from build123d import *

# Parameters (mm, degrees)
CROQUIS1_R                   = 25
CROQUIS1_R_2                 = 15
SALIENTE_EXTRUIR1_DEPTH      = 75
SALIENTE_EXTRUIR3_REACH      = 184.916
SALIENTE_EXTRUIR3_END_RADIUS = 25
SALIENTE_EXTRUIR3_START      = 100
CROQUIS2_R                   = 25
CROQUIS2_R_2                 = 15
CORTAR_EXTRUIR1_REACH        = 129.475
CROQUIS2_2_R                 = 15
SALIENTE_EXTRUIR4_REACH      = 164.475
SALIENTE_EXTRUIR4_END_RADIUS = 25
SALIENTE_EXTRUIR4_START      = 35
CROQUIS3_W                   = 35
CROQUIS3_H                   = 30
REDONDEO1_R                  = 15
CROQUIS4_R                   = 8
CORTAR_EXTRUIR2_DEPTH        = 151.7481344
SALIENTE_EXTRUIR5_START      = 55
SALIENTE_EXTRUIR5_DEPTH      = 10
SALIENTE_EXTRUIR6_START      = 22.912881
CROQUIS6_R                   = 10
CROQUIS6_R_2                 = 5
SALIENTE_EXTRUIR6_DEPTH      = 12.087119
CORTAR_EXTRUIR3_REACH        = 149.717
CROQUIS6_2_R                 = 5
REDONDEO1_OF_SIMETR_A1_R     = 15


with BuildPart() as part:
    # Croquis1 → Saliente-Extruir1 (new, symmetric)
    with BuildSketch(Plane.XY):
        Circle(CROQUIS1_R)
        Circle(CROQUIS1_R_2, mode=Mode.SUBTRACT)
    extrude(amount=SALIENTE_EXTRUIR1_DEPTH, both=True)

    # Saliente-Extruir3: up to this cylinder (the profile starts outside it)
    saliente_extruir3_end = Plane(origin=(0, 0, 24.292893), z_dir=(0, 0, -1)) * Cylinder(SALIENTE_EXTRUIR3_END_RADIUS, 420.832, mode=Mode.PRIVATE)
    # Croquis2 → Saliente-Extruir3 (add, up to the surface)
    with BuildSketch(Plane(origin=(0, 0, 0), x_dir=(0, 0, -1), z_dir=(1, 0, 0)).offset(SALIENTE_EXTRUIR3_START), mode=Mode.PRIVATE) as saliente_extruir3_sk1:
        Circle(CROQUIS2_R)
        Circle(CROQUIS2_R_2, mode=Mode.SUBTRACT)
    saliente_extruir3_tool1 = extrude(saliente_extruir3_sk1.sketch, amount=-SALIENTE_EXTRUIR3_REACH, mode=Mode.PRIVATE) - saliente_extruir3_end
    add(saliente_extruir3_tool1.solids().sort_by_distance((100, 0, 24.292893))[0])

    # Croquis2<2> → Cortar-Extruir1 (cut, up to next)
    with BuildSketch(Plane(origin=(0, 0, 0), x_dir=(0, 0, -1), z_dir=(1, 0, 0)), mode=Mode.PRIVATE) as cortar_extruir1_sk1:
        Circle(CROQUIS2_2_R)
    cortar_extruir1_tool1 = extrude(cortar_extruir1_sk1.sketch, amount=CORTAR_EXTRUIR1_REACH, mode=Mode.PRIVATE) & part.part
    add(cortar_extruir1_tool1.solids().sort_by_distance((0, 0, 0))[0], mode=Mode.SUBTRACT)

    # Saliente-Extruir4: up to this cylinder (the profile starts outside it)
    saliente_extruir4_end = Plane(origin=(82.5, 0, 0), z_dir=(1, 0, 0)) * Cylinder(SALIENTE_EXTRUIR4_END_RADIUS, 379.95, mode=Mode.PRIVATE)
    # Croquis3 → Saliente-Extruir4 (add, up to the surface)
    with BuildSketch(Plane.XY.offset(SALIENTE_EXTRUIR4_START), mode=Mode.PRIVATE) as saliente_extruir4_sk1:
        with Locations((82.5, 0)):
            Rectangle(CROQUIS3_W, CROQUIS3_H)
    saliente_extruir4_tool1 = extrude(saliente_extruir4_sk1.sketch, amount=-SALIENTE_EXTRUIR4_REACH, mode=Mode.PRIVATE) - saliente_extruir4_end
    saliente_extruir4 = saliente_extruir4_tool1.solids().sort_by_distance((82.5, 0, 35))[0]
    add(saliente_extruir4)

    # Redondeo1
    # the kernel refuses this fillet: 15 mm, written as the material it takes off along each edge
    with BuildSketch(Plane(origin=(65, 15, 72.5), x_dir=(1, 0, 0), z_dir=(0, 0, -1))) as redondeo1_piece_1_section:
        with BuildLine():
            CenterArc((REDONDEO1_R, REDONDEO1_R), REDONDEO1_R, 180, 90)
            Line((0, REDONDEO1_R), (0, 0))
            Line((0, 0), (REDONDEO1_R, 0))
        make_face()
    redondeo1_piece_1 = extrude(amount=90, mode=Mode.PRIVATE)
    redondeo1_piece_1 = redondeo1_piece_1 - Plane(origin=(68.454600716, 0, 0), x_dir=(0, 0, -1), z_dir=(1, 0, 0)) * Cylinder(25, 240, mode=Mode.PRIVATE)
    add(redondeo1_piece_1, mode=Mode.SUBTRACT)
    with BuildSketch(Plane(origin=(65, -15, 72.5), x_dir=(0, 1, 0), z_dir=(0, 0, -1))) as redondeo1_piece_2_section:
        with BuildLine():
            CenterArc((REDONDEO1_R, REDONDEO1_R), REDONDEO1_R, 180, 90)
            Line((0, REDONDEO1_R), (0, 0))
            Line((0, 0), (REDONDEO1_R, 0))
        make_face()
    redondeo1_piece_2 = extrude(amount=90, mode=Mode.PRIVATE)
    redondeo1_piece_2 = redondeo1_piece_2 - Plane(origin=(68.454600972, 0, 0), x_dir=(0, 0, -1), z_dir=(1, 0, 0)) * Cylinder(25, 240, mode=Mode.PRIVATE)
    add(redondeo1_piece_2, mode=Mode.SUBTRACT)

    # Croquis4 → Cortar-Extruir2 (cut, through all)
    with BuildSketch(Plane.XY.offset(35)):
        with Locations((80, 0)):
            Circle(CROQUIS4_R)
    cortar_extruir2 = extrude(amount=-CORTAR_EXTRUIR2_DEPTH, mode=Mode.SUBTRACT)

    # Croquis5 → Saliente-Extruir5 (add)
    with BuildSketch(Plane.XY.offset(SALIENTE_EXTRUIR5_START)):
        with BuildLine():
            ThreePointArc((-20.425558294, -14.415150654), (-17.67766953, 17.67766953), (14.415150654, 20.425558294))
            Line((14.415150654, 20.425558294), (-66.097829909, 77.246856773))
            ThreePointArc((-66.097829909, 77.246856773), (-76.367532368, 76.367532368), (-77.246856773, 66.097829909))
            Line((-77.246856773, 66.097829909), (-20.425558294, -14.415150654))
        make_face()
        with BuildLine():
            ThreePointArc((-74.246212025, 67.175144213), (-74.246212025, 74.246212025), (-67.175144213, 74.246212025))
            Line((-67.175144213, 74.246212025), (-31.819805153, 38.890872965))
            ThreePointArc((-31.819805153, 38.890872965), (-31.819805153, 31.819805153), (-38.890872965, 31.819805153))
            Line((-38.890872965, 31.819805153), (-74.246212025, 67.175144213))
        make_face(mode=Mode.SUBTRACT)
    saliente_extruir5 = extrude(amount=-SALIENTE_EXTRUIR5_DEPTH)

    # Croquis6 → Saliente-Extruir6 (add)
    with BuildSketch(Plane(origin=(0, 0, 0), x_dir=(1, 0, 0), z_dir=(0, 1, 0)).offset(SALIENTE_EXTRUIR6_START)):
        with Locations(Location((0, 0, 0), (0, 0, 270))):
            Circle(CROQUIS6_R)
        with Locations(Location((0, 0, 0), (0, 0, 270))):
            Circle(CROQUIS6_R_2, mode=Mode.SUBTRACT)
    extrude(amount=SALIENTE_EXTRUIR6_DEPTH)

    # Croquis6<2> → Cortar-Extruir3 (cut, up to next)
    with BuildSketch(Plane(origin=(0, 0, 0), x_dir=(1, 0, 0), z_dir=(0, 1, 0)), mode=Mode.PRIVATE) as cortar_extruir3_sk1:
        with Locations(Location((0, 0, 0), (0, 0, 270))):
            Circle(CROQUIS6_2_R)
    cortar_extruir3_tool1 = extrude(cortar_extruir3_sk1.sketch, amount=CORTAR_EXTRUIR3_REACH, mode=Mode.PRIVATE) & part.part
    add(cortar_extruir3_tool1.solids().sort_by_distance((0, 0, 0))[0], mode=Mode.SUBTRACT)

    # Simetría1: Saliente-Extruir4, Cortar-Extruir2, Saliente-Extruir5 across plane
    add(saliente_extruir4.mirror(Plane.XY))
    add(cortar_extruir2.mirror(Plane.XY), mode=Mode.SUBTRACT)
    add(saliente_extruir5.mirror(Plane.XY))

    # Redondeo1 of Simetría1
    # the kernel refuses this fillet: 15 mm, written as the material it takes off along each edge
    with BuildSketch(Plane(origin=(65, 15, -72.5), x_dir=(0, -1, 0), z_dir=(0, 0, 1))) as redondeo1_of_simetr_a1_piece_1_section:
        with BuildLine():
            CenterArc((REDONDEO1_OF_SIMETR_A1_R, REDONDEO1_OF_SIMETR_A1_R), REDONDEO1_OF_SIMETR_A1_R, 180, 90)
            Line((0, REDONDEO1_OF_SIMETR_A1_R), (0, 0))
            Line((0, 0), (REDONDEO1_OF_SIMETR_A1_R, 0))
        make_face()
    redondeo1_of_simetr_a1_piece_1 = extrude(amount=90, mode=Mode.PRIVATE)
    redondeo1_of_simetr_a1_piece_1 = redondeo1_of_simetr_a1_piece_1 - Plane(origin=(68.454600972, 0, 0), x_dir=(0, 0, -1), z_dir=(1, 0, 0)) * Cylinder(25, 240, mode=Mode.PRIVATE)
    add(redondeo1_of_simetr_a1_piece_1, mode=Mode.SUBTRACT)
    with BuildSketch(Plane(origin=(65, -15, -72.5), x_dir=(0, 1, 0), z_dir=(0, 0, 1))) as redondeo1_of_simetr_a1_piece_2_section:
        with BuildLine():
            CenterArc((REDONDEO1_OF_SIMETR_A1_R, -REDONDEO1_OF_SIMETR_A1_R), REDONDEO1_OF_SIMETR_A1_R, 90, 90)
            Line((0, -REDONDEO1_OF_SIMETR_A1_R), (0, 0))
            Line((0, 0), (REDONDEO1_OF_SIMETR_A1_R, 0))
        make_face()
    redondeo1_of_simetr_a1_piece_2 = extrude(amount=90, mode=Mode.PRIVATE)
    redondeo1_of_simetr_a1_piece_2 = redondeo1_of_simetr_a1_piece_2 - Plane(origin=(68.454600579, 0, 0), x_dir=(0, 0, -1), z_dir=(1, 0, 0)) * Cylinder(25, 240, mode=Mode.PRIVATE)
    add(redondeo1_of_simetr_a1_piece_2, mode=Mode.SUBTRACT)


solid = part.part
For this review, take the finished solid that the model builds, in its own axes (mm). A direction names the side the tool comes from. Round coordinates to 2 decimals unless told otherwise and drop trailing zeros. Order: outer loops, then holes, each group sorted by start corner. A loop starts at its lowest first (then second) coordinate and runs counter-clockwise, first axis right, second up. Notation, with made-up numbers: M -4,-40 L 11,-40 A18 ccw 11,-9 Z; hole C -27,9 d3. An arc over 180 degrees is marked long. Use a Markdown table: item, result. Add a question column.
Item 1: Add section B-B, the plane z = -51. Give the boundary of the cut face in (x, y), then the cut area to 3 significant figures.
Item 2: Add section D-D, the plane x = 37. Give the boundary of the cut face in (y, z).
Item 3: Add section C-C, the plane y = 60.5. Give the boundary of the cut face in (x, z).
Item 4: To check wall thickness, follow line 1 along Z through (x, y) = (-55, 68); line 2 along Y through (x, z) = (80, -25.75); line 3 along Z through (x, y) = (20, 0). State the ranges of each line that lie inside material, in increasing order.
Item 5: Tool access review of faces 1 (the flat face through (90, 0, -35)), 2 (the flat face through (90, 0, 35)), 3 (the cylindrical face through (65, 0, 29)), 4 (the flat face through (-25.28, 48.44, -50.07)): name each direction out of +Z, -Z, +X, -X, +Y, -Y from which nothing blocks a thin tool from reaching the whole face with its end or side.
Item 6: Mouldability with a two-part tool opening along Y and no side actions: class faces 5 (the flat face through (-56.32, 49.25, 50.07)), 6 (the flat face through (100, 0, -16)), 7 (the flat face through (90, 15, -28)) as released by +Y, released by -Y, zero draft, split by the parting line, or undercut.
Item 7: Add section A-A, the plane z = 31.5. Give the boundary of the cut face in (x, y).
Item 8: Insertion check: pin 1 (10 mm diameter, centred on x = 60, z = 16.5, fed in from -Y); pin 2 (2 mm diameter, centred on x = 28, y = -8.5, fed in from -Z); pin 3 (1 mm diameter, centred on x = -18.5, z = 52, fed in from -Y). Each pin has a flat end and moves straight along its axis. Give the tip position at first contact, or say it passes through.
Geometry results:
| question | item | result |
|---|---|---|
| 1 | outline | M -77.25,66.1 L -20.43,-14.42 A25 ccw long 14.42,20.43 L -66.1,77.25 A8 ccw Z; hole M -74.25,67.18 L -38.89,31.82 A5 ccw -31.82,38.89 L -67.18,74.25 A5 ccw Z; hole C 0,0 d30 |
| 1 | area | 3,140 mm² |
| 2 | outline | C 0,0 d50; hole C 0,0 d30 |
| 3 | outline | M -73.3,-55 L -67.57,-55 L -67.57,-45 L -73.3,-45 Z; M -73.3,45 L -67.57,45 L -67.57,55 L -73.3,55 Z; M -53.43,-55 L -42.37,-55 L -42.37,-45 L -53.43,-45 Z; M -53.43,45 L -42.37,45 L -42.37,55 L -53.43,55 Z |
| 4 | line 1 | z = -55 to -45, 45 to 55 |
| 4 | line 2 | y = -15 to -8, 8 to 15 |
| 4 | line 3 | z = -75 to -15, 15 to 75 |
| 5 | face 1 | -Z, +X, +Y, -Y |
| 5 | face 2 | +Z, +X, +Y, -Y |
| 5 | face 3 | +Z |
| 5 | face 4 | -Z, +X, +Y |
| 6 | face 5 | undercut |
| 6 | face 6 | zero draft |
| 6 | face 7 | released by +Y |
| 7 | outline | C 0,0 d50; M 80,-15 L 100,-15 L 100,15 L 80,15 A15 ccw Z; hole C 0,0 d30; hole C 80,0 d16 |
| 8 | pin 1 | stops at y = -22.2 |
| 8 | pin 2 | stops at z = -23.85 |
| 8 | pin 3 | stops at y = -17.35 |
